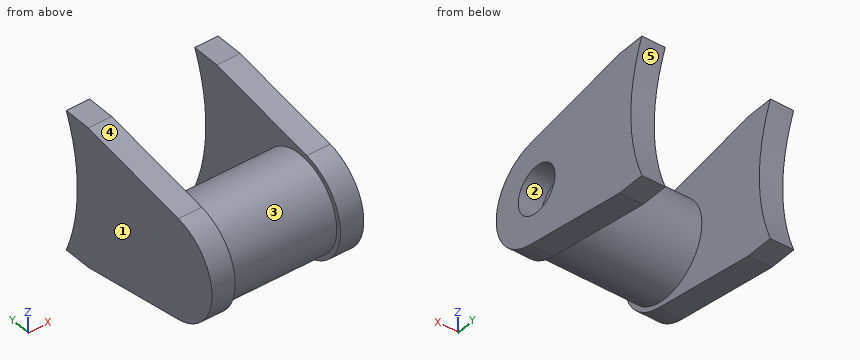
```python
from build123d import *

# Parameters (mm, degrees)
F0_R     = 12.7
F1_DEPTH = 14.2875
F2_R     = 12.7
F3_DEPTH = 6.35
F5_D     = 12.7
F5_DEPTH = 12.7
F5_TIP   = 3.8154649308


with BuildPart() as f1:
    # F0 (on Right) → F1 (new body, symmetric)
    with BuildSketch(Plane.YZ):
        with Locations((-25.6147123873, 0)):
            Circle(F0_R)
    extrude(amount=F1_DEPTH, both=True)

    # F2 (on face) → F3 (join)
    with BuildSketch(Plane.YZ.offset(14.2875)):
        with BuildLine():
            Line((10.7647620756, 19.05), (3.1447620756, 19.05))
            Line((3.1447620756, 19.05), (3.1447620756, -19.05))
            Line((3.1447620756, -19.05), (10.7647620756, -19.05))
            ThreePointArc((10.7647620756, -19.05), (6.9547620756, 0), (10.7647620756, 19.05))
        make_face()
        with BuildLine():
            Line((3.1447620756, -19.05), (3.1447620756, 19.05))
            Line((3.1447620756, 19.05), (-27.951915173, 13.7731036131))
            ThreePointArc((-27.951915173, 13.7731036131), (-16.6005519416, 10.672666558), (-11.6447123873, 0))
            ThreePointArc((-11.6447123873, 0), (-16.6005519416, -10.672666558), (-27.951915173, -13.7731036131))
            Line((-27.951915173, -13.7731036131), (3.1447620756, -19.05))
        make_face()
        with BuildLine():
            ThreePointArc((-11.6447123873, 0), (-16.6005519416, 10.672666558), (-27.951915173, 13.7731036131))
            ThreePointArc((-27.951915173, 13.7731036131), (-39.5847123873, 0), (-27.951915173, -13.7731036131))
            ThreePointArc((-27.951915173, -13.7731036131), (-16.6005519416, -10.672666558), (-11.6447123873, 0))
        make_face()
        with Locations((-25.6147123873, 0)):
            Circle(F2_R, mode=Mode.SUBTRACT)
        with Locations((-25.6147123873, 0)):
            Circle(F2_R)
    extrude(amount=F3_DEPTH)

    # F4: F1 across plane


with BuildPart() as f1_1:
    add(f1.part)
    add(f1.part.mirror(Plane.YZ))

    # F5 (one way)
    with BuildSketch(Plane(origin=(14.2875, 0, 0), x_dir=(0, 1, 0), z_dir=(-1, 0, 0))):
        with Locations((-25.6147123873, 0)):
            Circle(F5_D / 2)
    extrude(amount=-F5_DEPTH, mode=Mode.SUBTRACT)
    with Locations(Plane(origin=(14.2875, 0, 0), x_dir=(0, 1, 0), z_dir=(-1, 0, 0))):
        with Locations((-25.6147123873, 0)):
            with Locations((0, 0, -(F5_DEPTH + F5_TIP / 2))):  # 118° drill point
                Cone(0, F5_D / 2, F5_TIP, mode=Mode.SUBTRACT)


solid = f1_1.part
```
Model file for the job. Use its own axes, mm. Face numbers are marked on the shaded views. A direction names the side the tool comes from. Give positions to 0.01 mm unless a question says otherwise; leave off trailing zeros. Order: outer loops, then holes, each group sorted by start corner. A loop starts at its lowest first (then second) coordinate and runs counter-clockwise, first axis right, second up.
1) Saw through at B-B, the plane y = -11.5. Write the cut outline in (x, z), then the cut area to 3 significant figures.
2) Mould opens along Z. For the marked faces 3, 4 and 5 say: +Z half, -Z half, draft (parallel to the pull), parting line (faces both ways), or undercut.
3) Pin check, flat tips, straight feed: pin 1 (1.5 mm diameter, centred on x = -12.5, y = -24.5, fed in from +Z); pin 2 (12 mm diameter, centred on x = -1, y = -13.5, fed in from -Z); pin 3 (10 mm diameter, centred on x = -16, z = 13, fed in from -Y). Stop position of each tip, or through.
4) Saw through at A-A, the plane x = 18. Write the cut outline in (y, z).
5) Wall check: probe 1 along X at (y, z) = (7, -11); probe 2 along X at (y, z) = (-28.5, 4.5); probe 3 along Z at (x, y) = (14.5, -28). Give the ranges that are in metal, low to high.
6) Saw through at C-C, the plane z = 0. Write the cut outline in (x, y).
7) Saw through at D-D, the plane x = -8. Write the cut outline in (y, z).
8) 3-axis set-ups, long thin cutter, end or side, ignore diameter. For the marked faces 1 and 2: which of +Z, -Z, +X, -X, +Y, -Y reach the whole face in a straight line?
Computed:
1. outline: (-20.64, -16.56) - (-14.29, -16.56) - (-14.29, 16.56) - (-20.64, 16.56) - close; (14.29, -16.56) - (20.64, -16.56) - (20.64, 16.56) - (14.29, 16.56) - close
1. area: 421 mm2
2. face 3: parting line
2. face 4: +Z half
2. face 5: undercut
3. pin 1: stops at z = 12.69
3. pin 2: stops at z = -11.13
3. pin 3: stops at y = -37.07
4. outline: (-27.95, -13.77) - (3.14, -19.05) - (10.76, -19.05) arc R49.53 cw to (10.76, 19.05) - (3.14, 19.05) - (-27.95, 13.77) arc R13.97 ccw to start; hole circle Ø12.7 at (-25.61, 0)
5. probe 1: x = -20.64 to -14.29, 14.29 to 20.64
5. probe 2: x = -20.64 to 14.29
5. probe 3: z = -13.76 to -5.88, 5.88 to 13.76
6. outline: (-20.64, -39.58) - (-14.29, -39.58) - (-14.29, -38.31) - (14.29, -38.31) - (14.29, -39.58) - (20.64, -39.58) - (20.64, -31.96) - (14.29, -31.96) - (14.29, -19.26) - (20.64, -19.26) - (20.64, 6.95) - (14.29, 6.95) - (14.29, -12.91) - (-14.29, -12.91) - (-14.29, 6.95) - (-20.64, 6.95) - close
7. outline: circle Ø25.4 at (-25.61, 0)
8. face 1: +Z, -Z, -X, +Y, -Y
8. face 2: +X
